Autodesk Inventor part; units mm, degrees
ref_plane "YZ Plane" through (0, 0, 0) normal (1, 0, 0) x (0, 1, 0)
ref_plane "XZ Plane" through (0, 0, 0) normal (0, 1, 0) x (-1, 0, 0)
ref_plane "XY Plane" through (0, 0, 0) normal (0, 0, 1) x (1, 0, 0)
sketch "Sketch1" plane through (0, 0, 0) normal (0, 0, 1) x (1, 0, 0)
  line L0 (-17, -17) -> (17, -17)
  line L1 (17, -17) -> (17, 17)
  line L2 (17, 17) -> (-17, 17)
  line L3 (-17, 17) -> (-17, -17)
  line L4 (-17, -17) -> (17, 17) construction
  line L5 (17, -17) -> (-17, 17) construction
  line L6 (-17, -17) -> (-34, 0)
  line L7 (-34, 0) -> (-17, 17)
  point P0 (0, 0)
  point P1 (-17, 0)
  dimension "d154" = 34
  dimension "d155" = 34
  dimension "d180" = 17
extrude "Plate5" add sketch "Sketch1" along normal blind 2
fillet "Corner Round1" radius 2 5 edges at (17, 17, 1) (-17, 17, 1) (-17, -17, 1) (17, -17, 1) (-34, 0, 1)
properties part number "PRS 1200-52-03 FDS 1000 CUP 1" material "Stainless Steel"
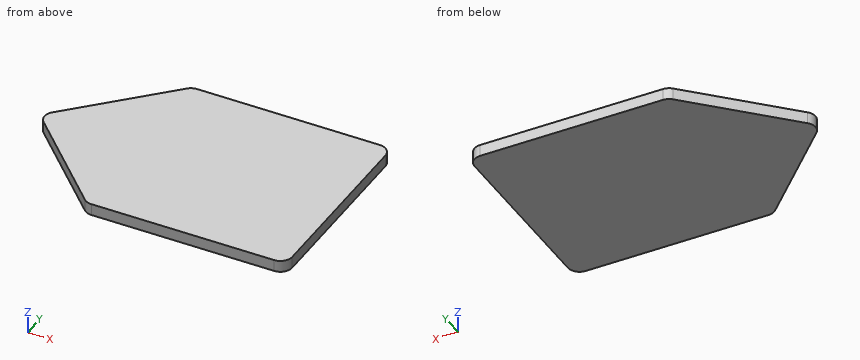
Here's how the part is built. I have some questions about the finished solid (model axes, mm). Give positions to 0.01 mm unless a question says otherwise; leave off trailing zeros. Order: outer loops, then holes, each group sorted by start corner. A loop starts at its lowest first (then second) coordinate and runs counter-clockwise, first axis right, second up. Notation, with made-up numbers: (75.25, -37) -> (102.25, -37) arc R15 cw to (102.25, -10) -> close; hole circle Ø7 at (66.5, -24.5). An arc over 180 degrees is marked (long way). Use CSV: the item, a comma, the result in double quotes. Start each with the question number.
Item 1: Suppose I cut it at C-C (x = -20.5). List the corners of the cut face in (y, z) for me.
Item 2: Suppose I cut it at B-B (y = -7). List the corners of the cut face in (x, z) for me.
Item 3: If I drill on probe 1 along Y at (x, z) = (-26, 0.2); probe 2 along X at (y, z) = (14, 0.7); probe 3 along Y at (x, z) = (-18, 0.35), over which ranges is the centre line in solid material (lowest first)? Write a range as [from, to].
Item 4: Suppose I cut it at A-A (z = 1.45). List the corners of the cut face in (x, y) for me, and give its area (3 significant figures).
Answer block:
1,outline,"(-13.5, 0) -> (13.5, 0) -> (13.5, 2) -> (-13.5, 2) -> close"
2,outline,"(-27, 0) -> (17, 0) -> (17, 2) -> (-27, 2) -> close"
3,probe 1,"y = [-8, 8]"
3,probe 2,"x = [-20, 17]"
3,probe 3,"y = [-16, 16]"
4,outline,"(-32.59, -1.41) -> (-17.59, -16.41) arc R2 ccw to (-16.17, -17) -> (15, -17) arc R2 ccw to (17, -15) -> (17, 15) arc R2 ccw to (15, 17) -> (-16.17, 17) arc R2 ccw to (-17.59, 16.41) -> (-32.59, 1.41) arc R2 ccw to start"
4,area,"1,440 mm^2"
